Work out the finished part from the listing and answer in its coordinate system (mm). A direction names the side the tool comes from. Coordinates: 2 decimals unless noted, no trailing zeros. Loops run counter-clockwise (first coordinate to the right, second up) from the corner with the lowest first, then second, coordinate; pieces in that order, holes last.
```python
from build123d import *

# Parameters (mm, degrees)
F0_R     = 40
F0_R_2   = 32.5
F1_DEPTH = 10
F2_W     = 20
F2_H     = 5
F3_DEPTH = 65


with BuildPart() as f1:
    # F0 (on Top) → F1 (new body)
    with BuildSketch(Plane.XY):
        Circle(F0_R)
        Circle(F0_R_2, mode=Mode.SUBTRACT)
    extrude(amount=-F1_DEPTH)

    # F2 (on Top) → F3 (join)
    with BuildSketch(Plane.XY):
        with Locations((0.680517, 35.432968)):
            Rectangle(F2_W, F2_H)
    extrude(amount=F3_DEPTH)


solid = f1.part
```
1. A cutting plane is placed at A-A, the plane x = 0. Give the vertices of the cut face in (y, z).
2. A cutting plane is placed at C-C, the plane z = 2. Give the vertices of the cut face in (x, y).
3. Determine the mould class of faces 5 (the cylindrical face through (31, 9.76, -4.93)), 6 (the flat face through (0, 33, -10)), 7 (the flat face through (1, 32.933, 32)), 8 (the cylindrical face through (-8.67, -39.05, -4.93)) for opening direction Y: released by +Y, released by -Y, zero draft, split by the parting line, or undercut.
4. A cutting plane is placed at B-B, the plane y = 0. Give the vertices of the cut face in (x, z), then the cut area to 3 significant figures.
5. For faces 1 (the flat face through (10.681, 35, 32)), 2 (the flat face through (1, 37.933, 32)), 3 (the flat face through (1, 35, 65)), 4 (the flat face through (-9.319, 35, 32)), determine the directions among +Z, -Z, +X, -X, +Y, -Y from which every point of the face is accessible in a straight line to the end or side of a thin tool.
6. A cutting plane is placed at D-D, the plane y = -11. Give the vertices of the cut face in (x, z).
7. Straight lines are drawn through the part: probe 1 along Y at (x, z) = (0, -3); probe 2 along Z at (x, y) = (-21.5, -29.5); probe 3 along X at (y, z) = (-17, -3). For each, find the intervals that lie inside material, in ascending order.
8. Each of these flat-tipped pins is pushed along its axis until it touches: P1, Ø22, axis at x = -1, z = 31, coming from the +Y side; P2, Ø4, axis at x = 17.5, z = 1, coming from the +Y side; P3, Ø6, axis at x = -3.5, z = 38.5, coming from the -Y side. Where does it stop, or does it pass through?
Answers below:
1. outline: (-40, -10) - (-32.5, -10) - (-32.5, 0) - (-40, 0) - close; (32.5, -10) - (40, -10) - (40, 0) - (37.93, 0) - (37.93, 65) - (32.93, 65) - (32.93, 0) - (32.5, 0) - close
2. outline: (-9.32, 32.93) - (10.68, 32.93) - (10.68, 37.93) - (-9.32, 37.93) - close
3. face 5: undercut
3. face 6: zero draft
3. face 7: released by -Y
3. face 8: split by the parting line
4. outline: (-40, -10) - (-32.5, -10) - (-32.5, 0) - (-40, 0) - close; (32.5, -10) - (40, -10) - (40, 0) - (32.5, 0) - close
4. area: 150 mm2
5. face 1: +Z, +X, +Y, -Y
5. face 2: +Z, +X, -X, +Y
5. face 3: +Z, +X, -X, +Y, -Y
5. face 4: +Z, -X, +Y, -Y
6. outline: (-38.46, -10) - (-30.58, -10) - (-30.58, 0) - (-38.46, 0) - close; (30.58, -10) - (38.46, -10) - (38.46, 0) - (30.58, 0) - close
7. probe 1: y = -40 to -32.5, 32.5 to 40
7. probe 2: z = -10 to 0
7. probe 3: x = -36.21 to -27.7, 27.7 to 36.21
8. P1: stops at y = 37.93
8. P2: stops at y = 36.76
8. P3: stops at y = 32.93
